```python
from build123d import *

# Parameters (mm, degrees)
SKETCH_W             = 507.5
SKETCH_H             = 64
PAD_DEPTH            = 15
POCKET_DEPTH         = 7.5
POCKET001_DEPTH      = 3.75
LINEARPATTERN_COUNT  = 5
LINEARPATTERN_PITCH  = 70.2
SKETCH003_W          = 15
SKETCH003_H          = 64
POCKET002_DEPTH      = 7.5
SKETCH004_R          = 1.5
POCKET003_DEPTH      = 15.001
POCKET003_DEPTH_BACK = 0.001
SKETCH005_R          = 1.5
POCKET004_DEPTH      = 20
SKETCH006_R          = 1.5
POCKET005_DEPTH      = 15.001


with BuildPart() as part:
    # Sketch → Pad (new body)
    with BuildSketch(Plane.YZ):
        with Locations((253.75, 32)):
            Rectangle(SKETCH_W, SKETCH_H)
    extrude(amount=PAD_DEPTH)

    # Sketch001 (on Face5 of Pad) → Pocket (cut)
    with BuildSketch(Plane(origin=(0, 0, 0), x_dir=(0, 1, 0), z_dir=(-1, 0, 0))):
        Polygon((0, -36.5), (507.5, -36.5), (507.5, -51.5), (0, -51.5), (0, -44), align=None)
    extrude(amount=-POCKET_DEPTH, mode=Mode.SUBTRACT)

    # Sketch002 (on Face4 of Pocket) → Pocket001 (cut)
    with BuildSketch(Plane(origin=(0, 0, 0), x_dir=(0, 1, 0), z_dir=(-1, 0, 0))):
        with BuildLine():
            Line((31.3, 0), (46.3, 0))
            Line((46.3, 0), (46.3, -34.5))
            ThreePointArc((46.3, -34.5), (46.885786, -35.914214), (48.3, -36.5))
            Line((29.3, -36.5), (48.3, -36.5))
            ThreePointArc((29.3, -36.5), (30.714214, -35.914214), (31.3, -34.5))
            Line((31.3, -34.5), (31.3, 0))
        make_face()
    pocket001 = extrude(amount=-POCKET001_DEPTH, mode=Mode.SUBTRACT)

    # LinearPattern: Pocket001 ×5
    with Locations(*[(0, i * LINEARPATTERN_PITCH, 0) for i in range(1, LINEARPATTERN_COUNT)]):
        add(pocket001, mode=Mode.SUBTRACT)

    # Sketch003 (on Face2 of MultiTransform) → Pocket002 (cut)
    with BuildSketch(Plane(origin=(0, 0, 0), x_dir=(0, 1, 0), z_dir=(-1, 0, 0))):
        with Locations((365.8, -32)):
            Rectangle(SKETCH003_W, SKETCH003_H)
    extrude(amount=-POCKET002_DEPTH, mode=Mode.SUBTRACT)

    # Sketch004 (on Face2 of Pocket002) → Pocket003 (cut, two sides)
    with BuildSketch(Plane(origin=(0, 0, 0), x_dir=(0, 1, 0), z_dir=(-1, 0, 0))) as pocket003_sk:
        with Locations((365.8, -10)):
            Circle(SKETCH004_R)
        with Locations((365.8, -31.5)):
            Circle(SKETCH004_R)
        with Locations((365.8, -56.5)):
            Circle(SKETCH004_R)
    extrude(amount=-POCKET003_DEPTH, mode=Mode.SUBTRACT)
    extrude(pocket003_sk.sketch, amount=POCKET003_DEPTH_BACK, mode=Mode.SUBTRACT)

    # Sketch005 (on Face29 of Pocket003) → Pocket004 (cut)
    with BuildSketch(Plane(origin=(0, 0, 0), x_dir=(0, 0, -1), z_dir=(0, -1, 0))):
        with Locations((-56.5, 7.5)):
            Circle(SKETCH005_R)
        with Locations((-31.5, 7.5)):
            Circle(SKETCH005_R)
        with Locations((-10, 7.5)):
            Circle(SKETCH005_R)
    extrude(amount=-POCKET004_DEPTH, mode=Mode.SUBTRACT)

    # Sketch006 (on Face2 of Pocket003) → Pocket005 (cut, through all)
    with BuildSketch(Plane(origin=(0, 0, 0), x_dir=(0, 1, 0), z_dir=(-1, 0, 0))):
        with Locations((15.65, -10)):
            Circle(SKETCH006_R)
        with Locations((15.65, -31.5)):
            Circle(SKETCH006_R)
        with Locations((15.65, -56.5)):
            Circle(SKETCH006_R)
        with Locations((342.75, -10)):
            Circle(SKETCH006_R)
        with Locations((342.75, -31.5)):
            Circle(SKETCH006_R)
        with Locations((342.75, -56.5)):
            Circle(SKETCH006_R)
    extrude(amount=-POCKET005_DEPTH, mode=Mode.SUBTRACT)


solid = part.part
```
Part model, mm, in its own coordinate system. Round coordinates to 2 decimals unless told otherwise and drop trailing zeros. Order: outer loops, then holes, each group sorted by start corner. A loop starts at its lowest first (then second) coordinate and runs counter-clockwise, first axis right, second up. Notation, with made-up numbers: M -33.5,-1.5 L 7.5,-1.5 A21 cw 7.5,21.5 Z; hole C 65,84 d6. An arc over 180 degrees is marked long. Put each result on its own line as item: value. Start each with the question number.
1. Slice it at B-B on y = 84.5. List the corners of the cut face in (x, z), then the cut area to 4 significant figures.
2. Slice it at A-A on z = 21. List the corners of the cut face in (x, y), then the cut area to 3 significant figures.
3. Drill centre lines: probe 1 along Y at (x, z) = (8.5, 56.5); probe 2 along Y at (x, z) = (9.5, 56.5); probe 3 along Y at (x, z) = (5.25, 56.5). Where is each one in solid material? Low to high. Write a range as [from, to].
4. Two-plate mould, pull along Y, no slides. Class faces 1 (the face through (3.75, 109, 18)), 2 (the face through (0, 439, 58)), 3 (the face through (3.75, 320, 18)), 4 (the face through (7, 507.5, 32)): +Y half, -Y half, draft (parallel to the pull), parting line (faces both ways), or undercut.
5. Drop flat-ended pins along their axis: pin 1 (4 mm diameter, centred on y = 437, z = 53.5, fed in from -X); pin 2 (5.5 mm diameter, centred on y = 36.5, z = 12, fed in from -X). Give the stop position or say it passes through.
Findings:
1. outline: M 0,0 L 15,0 L 15,64 L 0,64 L 0,51.5 L 7.5,51.5 L 7.5,36.5 L 0,36.5 Z
1. area: 847.5 mm2
2. outline: M 0,0 L 15,0 L 15,507.5 L 0,507.5 L 0,373.3 L 7.5,373.3 L 7.5,358.3 L 0,358.3 L 0,327.1 L 3.75,327.1 L 3.75,312.1 L 0,312.1 L 0,256.9 L 3.75,256.9 L 3.75,241.9 L 0,241.9 L 0,186.7 L 3.75,186.7 L 3.75,171.7 L 0,171.7 L 0,116.5 L 3.75,116.5 L 3.75,101.5 L 0,101.5 L 0,46.3 L 3.75,46.3 L 3.75,31.3 L 0,31.3 Z
2. area: 7,220 mm2
3. probe 1: [20, 341.25], [344.25, 364.3], [367.3, 507.5]
3. probe 2: [0, 14.15], [17.15, 341.25], [344.25, 364.3], [367.3, 507.5]
3. probe 3: [0, 14.15], [17.15, 341.25], [344.25, 358.3], [373.3, 507.5]
4. face 1: undercut
4. face 2: draft
4. face 3: undercut
4. face 4: +Y half
5. pin 1: x = 0
5. pin 2: x = 3.75
